Geometry check sheet. Reference: drawing and pictorial views, mm from the part's lowest x, y, z. Coordinates: 2 decimals unless noted, no trailing zeros. Loops run counter-clockwise (first coordinate to the right, second up) from the corner with the lowest first, then second, coordinate; pieces in that order, holes last. Notation, with made-up numbers: (41, 74) - (90, 74) arc R24 cw to (90, 102) - close; hole circle Ø6 at (-31.75, -37.75). An arc over 180 degrees is marked (long way). Write each question's results on one line, items separated by ' | '. Start each with the question number.
1. Cross-section at B-B (x = 44.2). Record the cut outline in (y, z), and give its area (3 significant figures).
2. Cross-section at C-C (z = 0.5). Give the number of separate pieces and of enclosed holes in the cut face, and give its area (3 significant figures).
3. Cross-section at A-A (y = 40.8). Record the cut outline in (x, z).
4. Thickness scan on line 1 (Y direction, x = 20.8, z = 0.3); line 2 (X direction, y = 76.5, z = 0.45); line 3 (Y direction, x = 9, z = 0.65). Record the ranges inside material, lowest first. Write a range as [from, to].
5. Gauge pin test, flat ends, axial feed: P1, Ø3.5, axis at x = 9.76, y = 76.5, coming from the +Z side; P2, Ø0.5, axis at x = 35, z = 0.5, coming from the -Y side. Record the tip position at first contact, or that the pin passes through.
6. Cross-section at D-D (y = 15.5). Record the cut outline in (x, z), and give its area (3 significant figures).
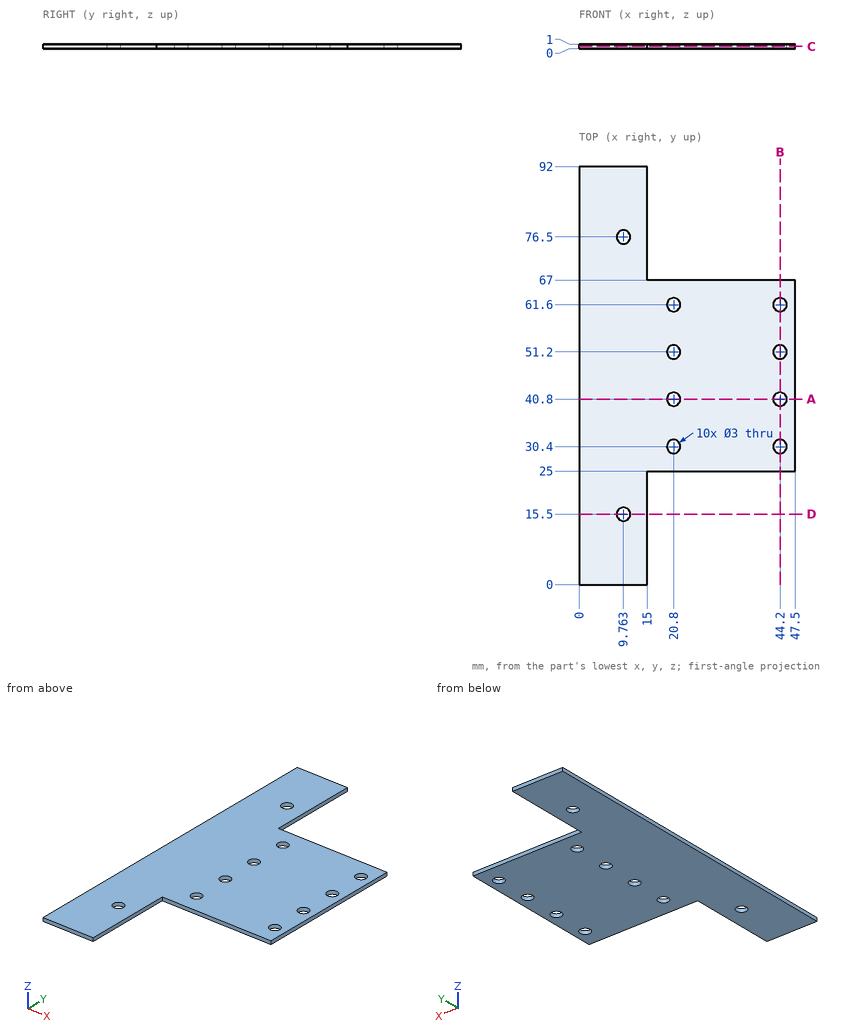
Established:
1) outline: (25, 0) - (28.9, 0) - (28.9, 1) - (25, 1) - close; (31.9, 0) - (39.3, 0) - (39.3, 1) - (31.9, 1) - close; (42.3, 0) - (49.7, 0) - (49.7, 1) - (42.3, 1) - close; (52.7, 0) - (60.1, 0) - (60.1, 1) - (52.7, 1) - close; (63.1, 0) - (67, 0) - (67, 1) - (63.1, 1) - close | area: 30.0 mm^2
2) separate pieces: 1 | enclosed holes: 10 | area: 2,670 mm^2
3) outline: (0, 0) - (19.3, 0) - (19.3, 1) - (0, 1) - close; (22.3, 0) - (42.7, 0) - (42.7, 1) - (22.3, 1) - close; (45.7, 0) - (47.5, 0) - (47.5, 1) - (45.7, 1) - close
4) line 1: [25, 28.9], [31.9, 39.3], [42.3, 49.7], [52.7, 60.1], [63.1, 67] | line 2: [0, 8.26], [11.26, 15] | line 3: [0, 14.21], [16.79, 75.21], [77.79, 92]
5) P1: z = 1 | P2: y = 25
6) outline: (0, 0) - (8.26, 0) - (8.26, 1) - (0, 1) - close; (11.26, 0) - (15, 0) - (15, 1) - (11.26, 1) - close | area: 12.0 mm^2
